```python
from build123d import *

# Parameters (mm, degrees)
SURFACE_EXTRUSION1_1_DEPTH = 30
EPAISSIR1_T1               = 2
EPAISSIR2_OUTLINE_W        = 50
EPAISSIR2_OUTLINE_H        = 20
EPAISSIR2_DEPTH            = 2
BOSS_EXTRU_1_DEPTH         = 17
BOSS_EXTRU_1_DEPTH_BACK    = 1
ESQUISSE2_W                = 44
ESQUISSE2_H                = 23
ESQUISSE3_W                = 11.316968607
ESQUISSE3_H                = 6
ENL_V_MAT_EXTRU_1_DEPTH    = 47


# Read off the part's stored shape, not the designer's step: Epaissir2
with BuildPart() as body_1:
    # Surface-Extrusion1: a surface, the sketch's curves swept straight by 30 mm
    with BuildLine(Plane(origin=(0, 0, 0), x_dir=(1, 0, 0), z_dir=(0, 1, 0)), mode=Mode.PRIVATE) as surface_extrusion1_1_path:
        Line((0, 0), (-50, 0))
        Line((-50, 0), (-50, 20))
        Line((-50, 20), (0, 20))
        Line((0, 20), (0, 0))
    surface_extrusion1_1 = Shell.extrude(surface_extrusion1_1_path.wire(), (0 * SURFACE_EXTRUSION1_1_DEPTH, 1 * SURFACE_EXTRUSION1_1_DEPTH, 0 * SURFACE_EXTRUSION1_1_DEPTH))
    add(Solid.thicken(surface_extrusion1_1, EPAISSIR1_T1))

    # Epaissir2 outline → Epaissir2 (add)
    with BuildSketch(Plane(origin=(0, 0, 0), x_dir=(1, 0, 0), z_dir=(0, 1, 0))):
        with Locations((-25, 10)):
            Rectangle(EPAISSIR2_OUTLINE_W, EPAISSIR2_OUTLINE_H)
    extrude(amount=EPAISSIR2_DEPTH)

    # Esquisse2 → Boss.-Extru.1 (add, two sides: drawn at the far end of the back side and taken through both)
    with BuildSketch(Plane(origin=(0, 0, -22), x_dir=(-1, 0, 0), z_dir=(0, 0, -1)).offset(-BOSS_EXTRU_1_DEPTH_BACK)):
        with Locations((20, 41.5)):
            Rectangle(ESQUISSE2_W, ESQUISSE2_H)
    extrude(amount=BOSS_EXTRU_1_DEPTH + BOSS_EXTRU_1_DEPTH_BACK)

    # Esquisse3 → Enlèv. mat.-Extru.1 (cut)
    with BuildSketch(Plane.ZY.offset(52)):
        with Locations((-33.341515696, 48)):
            Rectangle(ESQUISSE3_W, ESQUISSE3_H)
    extrude(amount=-ENL_V_MAT_EXTRU_1_DEPTH, mode=Mode.SUBTRACT)


solid = body_1.part
```
Verification items for the finished model (mm, model axes). A direction names the side the tool comes from. Give positions to 0.01 mm unless a question says otherwise; leave off trailing zeros. Order: outer loops, then holes, each group sorted by start corner. A loop starts at its lowest first (then second) coordinate and runs counter-clockwise, first axis right, second up. Notation, with made-up numbers: M -15.5,38 L 14.5,38 A25 ccw 14.5,50 Z; hole C -32,64.25 d1. An arc over 180 degrees is marked long. Answer in a Markdown table with one row per item. Add a question column.
Item 1: Tool access check on faces 1 (the flat face through (-25, 15, -22)), 2 (the flat face through (-24, 51, -33)), 3 (the flat face through (-25, 16, -20)). Record the directions out of +Z, -Z, +X, -X, +Y, -Y that give a thin tool (end or side, any length) a straight path to the whole face; none if there is none.
Item 2: Section check B-B, the plane y = 24.5. Enter the section's corners in (x, z), and give its area (3 significant figures).
Item 3: Gauge pin test, flat ends, axial feed: pin 1 (3 mm diameter, centred on y = 47.5, z = -32, fed in from -X); pin 2 (15 mm diameter, centred on x = -37, y = 21.5, fed in from -Z); pin 3 (3.5 mm diameter, centred on x = -18, z = -33, fed in from -Y); pin 4 (18.5 mm diameter, centred on x = -19, z = -30, fed in from -Y). Record the tip position at first contact, or that the pin passes through.
Item 4: Section check C-C, the plane z = -7.5. Enter the section's corners in (x, y), and give its area (3 significant figures).
Item 5: Section check D-D, the plane y = 46. Enter the section's corners in (x, z), and give its area (3 significant figures).
Item 6: Mould release check, pull along X, two halves, no side actions. Record for faces 4 (the flat face through (-5, 48, -33)), 5 (the flat face through (-25, 0, -10)), 6 (the flat face through (-50, 16, -10)): released by +X, released by -X, zero draft, split by the parting line, or undercut.
Item 7: Section check A-A, the plane x = -2. Enter the section's corners in (y, z), and give its area (3 significant figures).
Item 8: Scan lines: probe 1 along Z at (x, y) = (-45.5, 22.5); probe 2 along Y at (x, z) = (-12, -29.5); probe 3 along X at (y, z) = (27.5, -8.5). Record each from-to range of solid material in increasing order. Write a range as from..to.
Filled sheet:
| question | item | result |
|---|---|---|
| 1 | face 1 | -Z, +X, -X, -Y |
| 1 | face 2 | -Z, -X |
| 1 | face 3 | +Y |
| 2 | outline | M -52,-22 L 2,-22 L 2,2 L -52,2 Z; hole M -50,-20 L 0,-20 L 0,0 L -50,0 Z |
| 2 | area | 296 mm^2 |
| 3 | pin 1 | stops at x = -5 |
| 3 | pin 2 | stops at z = -22 |
| 3 | pin 3 | stops at y = 30 |
| 3 | pin 4 | stops at y = 0 |
| 4 | outline | M -52,0 L 2,0 L 2,30 L 0,30 L 0,2 L -50,2 L -50,30 L -52,30 Z |
| 4 | area | 220 mm^2 |
| 5 | outline | M -42,-27.68 L -5,-27.68 L -5,-39 L 2,-39 L 2,-21 L -42,-21 Z |
| 5 | area | 373 mm^2 |
| 6 | face 4 | released by -X |
| 6 | face 5 | zero draft |
| 6 | face 6 | undercut |
| 7 | outline | M 0,-22 L 30,-22 L 30,-39 L 53,-39 L 53,-21 L 30,-21 L 30,-20 L 2,-20 L 2,0 L 30,0 L 30,2 L 0,2 Z |
| 7 | area | 574 mm^2 |
| 8 | probe 1 | z = -22..-20, 0..2 |
| 8 | probe 2 | y = 30..45, 51..53 |
| 8 | probe 3 | x = -52..-50, 0..2 |
